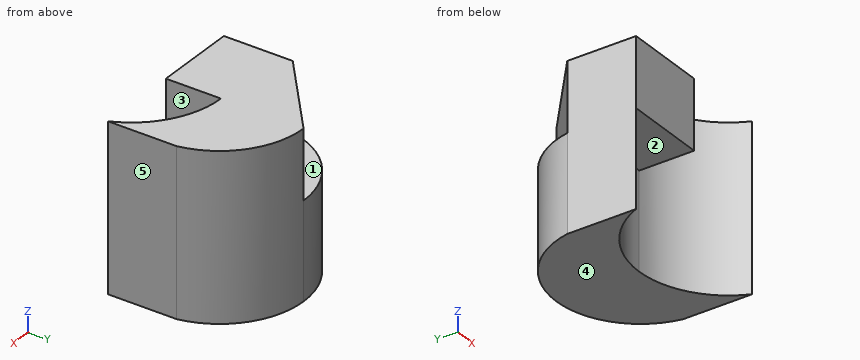
```python
from build123d import *

# Parameters (mm, degrees)
SKETCH1_W           = 6
SKETCH1_H           = 6
BOSS_EXTRUDE1_DEPTH = 5
CUT_EXTRUDE4_DEPTH  = 12.5
CUT_EXTRUDE5_DEPTH  = 2.5
CUT_EXTRUDE6_DEPTH  = 3.5


with BuildPart() as part:
    # Sketch1 → Boss-Extrude1 (new body)
    with BuildSketch(Plane(origin=(0, 0, 0), x_dir=(1, 0, 0), z_dir=(0, 1, 0))):
        Rectangle(SKETCH1_W, SKETCH1_H)
    extrude(amount=BOSS_EXTRUDE1_DEPTH)

    # Sketch5 → Cut-Extrude4 (cut)
    with BuildSketch(Plane.XY.offset(3)):
        with BuildLine():
            Line((-3, 5), (-3, 2.5))
            ThreePointArc((-3, 2.5), (-1.952562419, 4.293074903), (0, 5))
            Line((0, 5), (-3, 5))
        make_face()
        with BuildLine():
            ThreePointArc((0, 5), (1.952562419, 4.293074903), (3, 2.5))
            Line((3, 2.5), (3, 5))
            Line((3, 5), (0, 5))
        make_face()
        with BuildLine():
            ThreePointArc((3, 0), (1.802775638, 1.454163457), (0, 2))
            Line((0, 2), (0, 0))
            Line((0, 0), (3, 0))
        make_face()
    extrude(amount=-CUT_EXTRUDE4_DEPTH, mode=Mode.SUBTRACT)

    # Sketch6 → Cut-Extrude5 (cut)
    with BuildSketch(Plane.XY.offset(3)):
        with BuildLine():
            Line((-3, 2.5), (0, 5))
            ThreePointArc((0, 5), (-1.952562419, 4.293074903), (-3, 2.5))
        make_face()
    extrude(amount=-CUT_EXTRUDE5_DEPTH, mode=Mode.SUBTRACT)

    # Sketch7 → Cut-Extrude6 (cut)
    with BuildSketch(Plane(origin=(0, 0, -3), x_dir=(-1, 0, 0), z_dir=(0, 0, -1))):
        with BuildLine():
            Line((0, 2), (0, 0))
            Line((0, 0), (3, 0))
            ThreePointArc((3, 0), (1.802775638, 1.454163457), (0, 2))
        make_face()
    extrude(amount=-CUT_EXTRUDE6_DEPTH, mode=Mode.SUBTRACT)


solid = part.part
```
The listing builds one solid part. Answer for the finished solid, in the listing's coordinates (mm). Face numbers are marked on the shaded views. A direction names the side the tool comes from. Give positions to 0.01 mm unless a question says otherwise; leave off trailing zeros. Order: outer loops, then holes, each group sorted by start corner. A loop starts at its lowest first (then second) coordinate and runs counter-clockwise, first axis right, second up.
1) Find section D-D on y = 4. Write down the section's boundary in (x, z).
Reported:
outline: (-2.26, -3) - (2.26, -3) - (2.26, 3) - (-1.2, 3) - (-1.2, 0.5) - (-2.26, 0.5) - close
2) Find section A-A on y = 1.9. Write down the section's boundary in (x, z), then the cut area to 3 significant figures.
Reported:
outline: (-3, -3) - (-0.8, -3) - (-0.8, 0.5) - (0, 0.5) - (0, 3) - (-3, 3) - close; (0.8, -3) - (3, -3) - (3, 3) - (0.8, 3) - close
area: 28.4 mm2
3) Find section C-C on x = -0.5. Write down the section's boundary in (y, z).
Reported:
outline: (0, 0.5) - (1.96, 0.5) - (1.96, -3) - (4.96, -3) - (4.96, 0.5) - (4.58, 0.5) - (4.58, 3) - (0, 3) - close
4) For the marked faces 1, 2, 3, 4 and 5, determine the directions among +Z, -Z, +X, -X, +Y, -Y from which every point of the face is accessible in a straight line to the end or side of a thin tool.
Reported:
face 1: +Z, -X, +Y
face 2: -Z, -Y
face 3: +Z, -Z, -Y
face 4: -Z, +X, -X, +Y, -Y
face 5: +Z, -Z, +X, +Y, -Y
5) Find section B-B on z = 1.35. Write down the section's boundary in (x, y), then the cut area to 3 significant figures.
Reported:
outline: (-3, 0) - (0, 0) - (0, 2) arc R3.25 cw to (3, 0) - (3, 2.5) arc R3.05 ccw to (0, 5) - (-3, 2.5) - close
area: 20.1 mm2
6) Consider line 1 along X through (y, z) = (0.8, 1.4); line 2 along Z through (x, y) = (-1, 0.85); line 3 along Z through (x, y) = (-1, 4.8). Determine where each line is inside the solid, lowest interval first.
Reported:
line 1: x = -3 to 0, 2.52 to 3
line 2: z = 0.5 to 3
line 3: z = -3 to 0.5
7) Given P1, Ø1, axis at y = 4, z = -1, coming from the +X side; P2, Ø2, axis at y = 4.5, z = -1.5, coming from the -X side; P3, Ø1, axis at x = -1.5, y = 0.5, coming from the -Z side, each flat-ended and moving along its own axis, determine where each tip first touches the part or whether it passes through.
Reported:
P1: stops at x = 2.63
P2: stops at x = -2.63
P3: stops at z = 0.5
